Input: part model. Units: mm. Frame: model coordinates. A direction names the side the tool comes from. Coordinates: 2 decimals unless noted, no trailing zeros. Order: outer loops, then holes, each group sorted by start corner. A loop starts at its lowest first (then second) coordinate and runs counter-clockwise, first axis right, second up. Notation, with made-up numbers: (67, 13.25) - (99, 13.25) arc R25 ccw to (99, 26.25) - close; hole circle Ø5 at (3.25, -7). An arc over 180 degrees is marked (long way). Answer as CSV lines item,"result". Start each with the question number.
Item 1: Material intervals for line 1 along Y through (x, z) = (15.75, 431.5); line 2 along X through (y, z) = (35.5, 349); line 3 along X through (y, z) = (50.55, 215.9), sorted ascending.
Item 2: Access query for faces 5 (the flat face through (13, 1.27, 225)), 6 (the flat face through (0.4, 25.5, 457.2)). Directions: +Z, -Z, +X, -X, +Y, -Y. A direction counts if a zero-diameter tool reaches every point of the face in a straight line with its end or side. Return the directions, or none.
Item 3: Section B-B (x = 6.5). Output: boundary loops of the cut face in (y, z).
Item 4: Section A-A (y = 32). Output: boundary loops of the cut face in (x, z), and give its area (3 significant figures).
Item 5: Draft query along X for faces 1 (the flat face through (0.4, 25.5, 0)), 2 (the flat face through (13, 49.53, 225)), 3 (the flat face through (24.13, 25, 225)), 4 (the flat face through (25.4, 25, 225)). Return one class per face: +X half, -X half, draft (parallel to the pull), parting line (faces both ways), or undercut.
Item 6: Section C-C (z = 384). Output: boundary loops of the cut face in (x, y).
Autodesk Inventor part; units mm, degrees
ref_plane "YZ Plane" through (0, 0, 0) normal (1, 0, 0) x (0, 1, 0)
ref_plane "XZ Plane" through (0, 0, 0) normal (0, 1, 0) x (-1, 0, 0)
ref_plane "XY Plane" through (0, 0, 0) normal (0, 0, 1) x (1, 0, 0)
sketch "Sketch1" plane through (0, 0, 0) normal (0, 0, 1) x (1, 0, 0)
  line L0 (0, 0) -> (25.4, 0)
  line L1 (25.4, 0) -> (25.4, 50.8)
  line L2 (25.4, 50.8) -> (0, 50.8)
  line L3 (0, 50.8) -> (0, 0)
  line L4 (1.27, 1.27) -> (24.13, 1.27)
  line L5 (24.13, 1.27) -> (24.13, 49.53)
  line L6 (24.13, 49.53) -> (1.27, 49.53)
  line L7 (1.27, 49.53) -> (1.27, 1.27)
  dimension "d0" = 25.4
  dimension "d1" = 50.8
  dimension "d4" = 1.27
  dimension "d5" = 1.27
extrude "Extrusion1" add sketch "Sketch1" along normal blind 457.2
sketch "Sketch2" plane through (0, 50.8, 0) normal (0, 1, 0) x (1, 0, 0)
  line L0 (1.27, -457.2) -> (24.13, -457.2)
  circle A0 centre (12.7, -12.7) radius 2.0701
  line L1 (0, 0) -> (0, -457.2)
  line L2 (25.4, 0) -> (0, 0)
  dimension "d9" = 4.1402
  dimension "d10" = 12.7
  dimension "d11" = 12.7
extrude "Extrusion2" cut sketch "Sketch2" against normal blind 457.2
pattern_linear "Rectangular Pattern1" count 18 spacing 25.4 along (0, 0, 1) of "Extrusion2"
equation "\"d0\" = u1"
equation "\"d1\" = u2"
equation "\"d4\" = u3"
equation "\"d5\" = u3"
equation "\"d6\" = u4"
equation "\"d9\" = u5"
equation "\"d10\" = u6"
equation "\"d11\" = u7"
equation "\"d12\" = u4"
equation "\"d16\" = u9"
equation "\"u1\" = 25.4"
equation "\"u2\" = 50.8"
equation "\"u3\" = 1.27"
equation "\"u4\" = 457.2"
equation "\"u5\" = 4.1402"
equation "\"u6\" = 12.7"
equation "\"u7\" = 12.7"
equation "\"u9\" = 25.4"
properties part number "18in VerseFrame Uptake"
Determined:
1,line 1,"y = 0 to 1.27, 49.53 to 50.8"
1,line 2,"x = 0 to 1.27, 24.13 to 25.4"
1,line 3,"x = 0 to 10.63, 14.77 to 25.4"
2,face 5,"+Z, -Z"
2,face 6,"+Z, +X, -X, +Y, -Y"
3,outline,"(0, 0) - (1.27, 0) - (1.27, 457.2) - (0, 457.2) - close; (49.53, 0) - (50.8, 0) - (50.8, 457.2) - (49.53, 457.2) - close"
4,outline,"(0, 0) - (1.27, 0) - (1.27, 457.2) - (0, 457.2) - close; (24.13, 0) - (25.4, 0) - (25.4, 457.2) - (24.13, 457.2) - close"
4,area,"1,160 mm^2"
5,face 1,"draft"
5,face 2,"undercut"
5,face 3,"undercut"
5,face 4,"+X half"
6,outline,"(0, 0) - (25.4, 0) - (25.4, 50.8) - (0, 50.8) - close; hole (1.27, 1.27) - (24.13, 1.27) - (24.13, 49.53) - (1.27, 49.53) - close"
